```python
from build123d import *

# Parameters (mm, degrees)
SKETCH_W        = 62
SKETCH_H        = 24
PAD_DEPTH       = 62
SKETCH001_W     = 58
SKETCH001_H     = 20
POCKET_DEPTH    = 60
SKETCH002_W     = 8
SKETCH002_H     = 12
POCKET001_DEPTH = 2


with BuildPart() as part:
    # Sketch → Pad (new body)
    with BuildSketch(Plane.XY):
        with Locations((31, 12)):
            Rectangle(SKETCH_W, SKETCH_H)
    extrude(amount=PAD_DEPTH)

    # Sketch001 (on Face6 of Pad) → Pocket (cut)
    with BuildSketch(Plane.XY.offset(62)):
        with Locations((31, 12)):
            Rectangle(SKETCH001_W, SKETCH001_H)
    extrude(amount=-POCKET_DEPTH, mode=Mode.SUBTRACT)

    # Sketch002 (on Face1 of Pocket) → Pocket001 (cut)
    with BuildSketch(Plane.XZ):
        with Locations((49, 48)):
            Rectangle(SKETCH002_W, SKETCH002_H)
    extrude(amount=-POCKET001_DEPTH, mode=Mode.SUBTRACT)


solid = part.part
```
CAD build for the part. Positions are in the model's coordinates, mm. A direction names the side the tool comes from. Give positions to 0.01 mm unless a question says otherwise; leave off trailing zeros. Order: outer loops, then holes, each group sorted by start corner. A loop starts at its lowest first (then second) coordinate and runs counter-clockwise, first axis right, second up. Notation, with made-up numbers: M 58,49 L 84,49 A22 ccw 84,88 Z; hole C 43.25,42 d4. An arc over 180 degrees is marked long. Put each result on its own line as item: value. Start each with the question number.
(1) Mould opens along X. For faces 4 (the flat face through (31, 2, 32)), 5 (the flat face through (0, 12, 31)), 6 (the flat face through (31, 12, 0)), 7 (the flat face through (62, 12, 31)) say: +X half, -X half, draft (parallel to the pull), parting line (faces both ways), or undercut.
(2) Saw through at D-D, the plane x = 57.5. Write the cut outline in (y, z), then the cut area to 3 significant figures.
(3) Saw through at C-C, the plane z = 23.5. Write the cut outline in (x, y), then the cut area to 3 significant figures.
(4) Drill centre lines: line 1 along X through (y, z) = (5, 36); line 2 along Y through (x, z) = (53.5, 28.5); line 3 along Z through (x, y) = (35.5, 3.25). Where is each one in solid material? Low to high.
(5) Saw through at A-A, the plane x = 48. Write the cut outline in (y, z), then the cut area to 3 significant figures.
(6) Which spindle directions (+Z, -Z, +X, -X, +Y, -Y) get a long thin tool onto all of the face, cutting with end or side? Do faces 1 (the flat face through (29, 1, 62)), 2 (the flat face through (2, 12, 32)), 3 (the flat face through (45, 1, 48)). Say none if no direction does.
(7) Saw through at B-B, the plane y = 20.75. Write the cut outline in (x, z).
(8) Flat gauge pin, fed straight in: pin 1 Ø4 at (x, y) = (54.5, 4.5) entering from +Z. Where does the tip first touch, or does it go through?
Check result:
1. face 4: undercut
1. face 5: -X half
1. face 6: draft
1. face 7: +X half
2. outline: M 0,0 L 24,0 L 24,62 L 22,62 L 22,2 L 2,2 L 2,62 L 0,62 Z
2. area: 288 mm2
3. outline: M 0,0 L 62,0 L 62,24 L 0,24 Z; hole M 2,2 L 60,2 L 60,22 L 2,22 Z
3. area: 328 mm2
4. line 1: x = 0 to 2, 60 to 62
4. line 2: y = 0 to 2, 22 to 24
4. line 3: z = 0 to 2
5. outline: M 0,0 L 24,0 L 24,62 L 22,62 L 22,2 L 2,2 L 2,42 L 0,42 Z; M 0,54 L 2,54 L 2,62 L 0,62 Z
5. area: 264 mm2
6. face 1: +Z, +X, -X, +Y, -Y
6. face 2: +Z
6. face 3: -Y
7. outline: M 0,0 L 62,0 L 62,62 L 60,62 L 60,2 L 2,2 L 2,62 L 0,62 Z
8. pin 1: stops at z = 2
